Autodesk Inventor part; units mm, degrees
ref_plane "YZ Plane" through (0, 0, 0) normal (1, 0, 0) x (0, 1, 0)
ref_plane "XZ Plane" through (0, 0, 0) normal (0, 1, 0) x (-1, 0, 0)
ref_plane "XY Plane" through (0, 0, 0) normal (0, 0, 1) x (1, 0, 0)
sketch "Sketch1" plane through (0, 0, 0) normal (0, 1, 0) x (-1, 0, 0)
  line L0 (0, 0) -> (50.8, 0)
  line L1 (50.8, 0) -> (50.8, -101.6)
  line L2 (50.8, -101.6) -> (0, -101.6)
  line L3 (0, -101.6) -> (0, 0)
  dimension "d0" = 50.8
  dimension "d1" = 101.6
extrude "Extrusion1" add sketch "Sketch1" along normal blind 3.175
sketch "Sketch2" plane through (0, 0, 0) normal (0, -1, 0) x (1, 0, 0)
  line L0 (-50.8, 0) -> (0, 0)
  line L1 (0, 0) -> (3.175, 0)
  line L2 (3.175, 0) -> (3.175, 3.175)
  line L3 (3.175, 3.175) -> (0, 3.175)
  line L4 (0, 3.175) -> (0, 0)
  line L5 (0, -101.6) -> (-50.8, -101.6)
  line L6 (-50.8, -101.6) -> (-53.975, -101.6)
  line L7 (-53.975, -101.6) -> (-53.975, -104.775)
  line L8 (-53.975, -104.775) -> (-50.8, -104.775)
  line L9 (-50.8, -104.775) -> (-50.8, -101.6)
  line L10 (3.175, 3.175) -> (-53.975, 3.175)
  line L11 (-53.975, 3.175) -> (-53.975, -104.775)
  line L12 (-53.975, -104.775) -> (3.175, -104.775)
  line L13 (3.175, -104.775) -> (3.175, 3.175)
  line L14 (-50.8, -101.6) -> (0, -101.6)
  line L15 (0, -101.6) -> (0, 0)
  line L16 (0, 0) -> (-50.8, 0)
  line L17 (-50.8, 0) -> (-50.8, -101.6)
  dimension "d4" = 3.175
  dimension "d5" = 3.175
  dimension "d6" = 3.175
  dimension "d7" = 3.175
extrude "Extrusion2" add sketch "Sketch2" against normal blind 41.275 contours L17 L6 L11 L10 L4 L0 | L4 L3 L2 L1 | L1 L13 L12 L9 L5 L15 | L9 L8 L7 L6
sketch "Sketch3" plane through (0, 0, 0) normal (0, -1, 0) x (1, 0, 0)
  line L0 (0, -101.6) -> (0, 0)
  line L1 (3.175, 3.175) -> (3.175, -104.775)
  line L2 (0, 0) -> (3.175, 0)
  line L3 (3.175, 0) -> (12.065, 0)
  line L4 (12.065, 0) -> (12.065, -8.89)
  line L5 (12.065, -8.89) -> (3.175, -8.89)
  line L6 (3.175, -8.89) -> (3.175, 0)
  line L7 (-53.975, -104.775) -> (-53.975, 3.175)
  line L8 (-53.975, 0) -> (-62.865, 0)
  line L9 (-62.865, 0) -> (-62.865, -8.89)
  line L10 (-62.865, -8.89) -> (-53.975, -8.89)
  line L11 (-53.975, -8.89) -> (-53.975, 0)
  line L12 (-53.975, -101.6) -> (-62.865, -101.6)
  line L13 (-62.865, -101.6) -> (-62.865, -92.71)
  line L14 (-62.865, -92.71) -> (-53.975, -92.71)
  line L15 (-53.975, -92.71) -> (-53.975, -101.6)
  line L16 (3.175, -101.6) -> (12.065, -101.6)
  line L17 (12.065, -101.6) -> (12.065, -92.71)
  line L18 (12.065, -92.71) -> (3.175, -92.71)
  line L19 (3.175, -92.71) -> (3.175, -101.6)
  dimension "d11" = 8.89
  dimension "d12" = 8.89
  dimension "d13" = 8.89
  dimension "d14" = 8.89
  dimension "d15" = 8.89
  dimension "d16" = 8.89
  dimension "d17" = 8.89
  dimension "d18" = 8.89
extrude "Extrusion3" add sketch "Sketch3" against normal blind 3.175
fillet "Fillet1" radius 3.175 16 edges at (3.175, 1.5875, 0) (12.065, 1.5875, 0) (12.065, 1.5875, -8.89) (3.175, 1.5875, -8.89) (12.065, 1.5875, -92.71) (3.175, 1.5875, -92.71) (12.065, 1.5875, -101.6) (3.175, 1.5875, -101.6) (-53.975, 1.5875, -101.6) (-62.865, 1.5875, -101.6) (-62.865, 1.5875, -92.71) (-53.975, 1.5875, -92.71) (-53.975, 1.5875, 0) (-62.865, 1.5875, 0) (-62.865, 1.5875, -8.89) (-53.975, 1.5875, -8.89)
sketch "Sketch4" plane through (0, 3.175, 0) normal (0, 1, 0) x (1, 0, 0)
  line L0 (-59.69, 8.89) -> (-57.15, 8.89) construction
  line L1 (-58.42, 8.89) -> (-58.42, 0) construction
  line L2 (-59.69, 0) -> (-57.15, 0) construction
  line L3 (6.35, 8.89) -> (8.89, 8.89) construction
  line L4 (7.62, 8.89) -> (7.62, 0) construction
  line L5 (8.89, 0) -> (6.35, 0) construction
  line L6 (8.89, 101.6) -> (6.35, 101.6) construction
  line L7 (7.62, 101.6) -> (7.62, 92.71) construction
  line L8 (6.35, 92.71) -> (8.89, 92.71) construction
  line L9 (-57.15, 101.6) -> (-59.69, 101.6) construction
  line L10 (-58.42, 101.6) -> (-58.42, 92.71) construction
  line L11 (-59.69, 92.71) -> (-57.15, 92.71) construction
  point P0 (0, 0)
  point P1 (-58.42, 97.155)
  point P2 (7.62, 97.155)
  point P3 (7.62, 4.445)
  point P4 (-58.42, 4.445)
hole "Hole1" at (-58.42, 3.175, -97.155) at (7.62, 3.175, -97.155) at (7.62, 3.175, -4.445) at (-58.42, 3.175, -4.445) direction (0, -1, 0) diameter 3.175 depth 25.4 tip angle 118
sketch "Sketch5" plane through (0, 41.275, 0) normal (0, 1, 0) x (1, 0, 0)
  line L0 (-53.975, 104.775) -> (3.175, 104.775)
  line L1 (3.175, 104.775) -> (-9.525, 104.775)
  arc A0 (3.175, 104.775) -> (6.35, 101.6) centre (6.35, 104.775) ccw
  line L2 (3.175, 104.775) -> (3.175, 92.075)
  line L3 (3.175, 92.075) -> (-9.525, 104.775)
  line L4 (3.175, -3.175) -> (-53.975, -3.175)
  line L5 (3.175, -3.175) -> (3.175, 9.525)
  line L6 (3.175, -3.175) -> (3.175, 12.065)
  line L7 (3.175, -3.175) -> (-9.525, -3.175)
  line L8 (-9.525, -3.175) -> (3.175, 9.525)
  line L9 (-25.4, 104.775) -> (-25.4, -3.175) construction
  line L10 (3.175, 104.775) -> (-53.975, 104.775)
  line L11 (-53.975, 104.775) -> (-41.275, 104.775)
  line L12 (-53.975, 104.775) -> (-53.975, 92.075)
  line L13 (-53.975, 92.075) -> (-41.275, 104.775)
  line L14 (-53.975, -3.175) -> (3.175, -3.175)
  line L15 (-53.975, -3.175) -> (-53.975, 9.525)
  line L16 (-53.975, -3.175) -> (-41.275, -3.175)
  line L17 (-41.275, -3.175) -> (-53.975, 9.525)
  point P0 (0, 0)
  dimension "d29" = 12.7
  dimension "d30" = 12.7
  dimension "d31" = 12.7
  dimension "d32" = 12.7
extrude "Extrusion4" add sketch "Sketch5" against normal blind 39.37
fillet "Fillet2" radius 3.175 8 edges at (-6.35, 22.225, -101.6) (0, 22.225, -95.25) (-44.45, 22.225, -101.6) (-50.8, 22.225, -95.25) (-50.8, 22.225, -6.35) (-44.45, 22.225, 0) (-6.35, 22.225, 0) (0, 22.225, -6.35)
sketch "Sketch6" plane through (0, 41.275, 0) normal (0, 1, 0) x (1, 0, 0)
  line L0 (-50.8, 93.9349) -> (-50.8, 7.6651)
  line L1 (0, 0) -> (0, 93.9349)
  point P0 (-50.8, 0)
  point P1 (-50.8, 101.6)
  point P2 (-50.8, 101.6)
  point P3 (0, 101.6)
hole "Hole2" at (0, 41.275, 0) at (-50.8, 41.275, 0) at (-50.8, 41.275, -101.6) at (0, 41.275, -101.6) direction (0, -1, 0) diameter 3.175 depth 9.525 tip angle 118
sketch "Sketch7" plane through (-53.975, 41.275, 3.175) normal (0, 0, 1) x (1, 0, 0)
  line L0 (46.3099, -38.1) -> (10.8401, -38.1) construction
  line L1 (28.575, -38.1) -> (28.575, -31.75) construction
  line L2 (28.575, -31.75) -> (25.4, -31.75) construction
  line L3 (28.575, -31.75) -> (31.75, -31.75) construction
  circle A0 centre (25.4, -31.75) radius 3.175
  circle A1 centre (31.75, -31.75) radius 3.175
  line L4 (25.4, -28.575) -> (31.75, -28.575)
  line L5 (25.4, -34.925) -> (31.75, -34.925)
  point P0 (53.975, -41.275)
  dimension "d49" = 6.35
  dimension "d50" = 3.175
  dimension "d51" = 3.175
  dimension "d52" = 6.35
  dimension "d53" = 6.35
extrude "Extrusion5" cut sketch "Sketch7" against normal blind 25.4
properties part number "box"
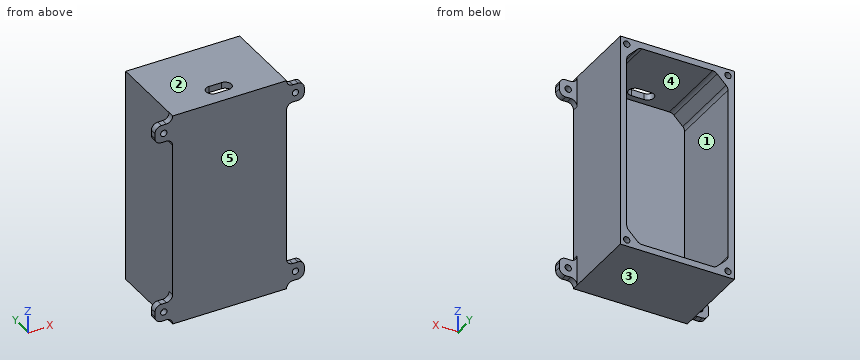
Geometry: final body of the model. Coordinates: model frame, mm. Face numbers are marked on the shaded views. A direction names the side the tool comes from. Round coordinates to 2 decimals unless told otherwise and drop trailing zeros. Write each loop counter-clockwise with the first axis right and the second up, starting at its lowest first coordinate (ties: lowest second). Pieces come first, ordered by that corner, then holes. Notation, with made-up numbers: (-8, 12.5) -> (47, 12.5) arc R15 ccw to (47, 31.5) -> close; hole circle Ø10 at (12, 24.25). An arc over 180 degrees is marked (long way). Use CSV: the item, a comma, the result in double quotes. Start each with the question number.
Q1. Pull-direction query (Z, two-part tool) for the marked faces 1, 2 and 3; classes: pulls with the +Z half, pulls with the -Z half, needs draft (parallel to the pull), parting line crosses it, or undercut.
Q2. Reachability of the marked faces 4 and 5 from +Z, -Z, +X, -X, +Y, -Y: full face, straight path, thin tool, end or side. Return the list, or none.
Q3. Section C-C (z = -20.5). Return loops of the section in (x, y) (3 decimals).
Q4. Section D-D (x = -38.5). Return loops of the section in (y, z) (3 decimals).
Q5. Section A-A (x = -58.42). Return loops of the section in (y, z) (1 decimal), plus the area to 3 significant figures.
Q6. Section B-B (y = 28). Return loops of the section in (x, z) (3 decimals).
Q7. Line query: L1, parallel to Z at x = 7.62, y = 0.7; L2, parallel to Z at x = -15, y = 8.5 (3 decimals); L3, parallel to X at y = 10.5, z = -72.5 (3 decimals). Output: solid intervals per line, ascending.
Q8. First-contact query: pin 1 Ø3 at (y, z) = (13, -65) entering from +X (3 decimals); pin 2 Ø2 at (x, y) = (7, 2) entering from -Z; pin 3 Ø5 at (x, z) = (7.62, -97.155) entering from +Y (3 decimals). Flat tips, straight axial feed; report the tip coordinate or a pass-through.
Result sheet:
1,face 1,"undercut"
1,face 2,"pulls with the +Z half"
1,face 3,"pulls with the -Z half"
2,face 4,"+Y"
2,face 5,"+Z, -Z, +X, -X, -Y"
3,outline,"(-53.975, 0) -> (3.175, 0) -> (3.175, 41.275) -> (0, 41.275) -> (0, 3.175) -> (-50.8, 3.175) -> (-50.8, 41.275) -> (-53.975, 41.275) -> close"
4,outline,"(0, -104.775) -> (41.275, -104.775) -> (41.275, -101.6) -> (3.175, -101.6) -> (3.175, 0) -> (41.275, 0) -> (41.275, 3.175) -> (0, 3.175) -> close"
5,outline,"(0, -101.6) -> (3.2, -101.6) -> (3.2, -98.7) -> (0, -98.7) -> close; (0, -95.6) -> (3.2, -95.6) -> (3.2, -92.7) -> (0, -92.7) -> close; (0, -8.9) -> (3.2, -8.9) -> (3.2, -6) -> (0, -6) -> close; (0, -2.9) -> (3.2, -2.9) -> (3.2, 0) -> (0, 0) -> close"
5,area,"36.3 mm²"
6,outline,"(-53.975, -104.775) -> (3.175, -104.775) -> (3.175, 3.175) -> (-53.975, 3.175) -> close; hole (-50.8, -93.935) arc R3.175 ccw to (-49.87, -96.18) -> (-45.38, -100.67) arc R3.175 ccw to (-43.135, -101.6) -> (-7.665, -101.6) arc R3.175 ccw to (-5.42, -100.67) -> (-0.93, -96.18) arc R3.175 ccw to (0, -93.935) -> (0, -7.665) arc R3.175 ccw to (-0.93, -5.42) -> (-5.42, -0.93) arc R3.175 ccw to (-7.665, 0) -> (-43.135, 0) arc R3.175 ccw to (-45.38, -0.93) -> (-49.87, -5.42) arc R3.175 ccw to (-50.8, -7.665) -> close"
7,L1,"-101.6 to -98.74, -95.57 to -92.71, -8.89 to -6.03, -2.86 to 0"
7,L2,"-104.775 to -101.6, 0 to 3.175"
7,L3,"-53.975 to -50.8, 0 to 3.175"
8,pin 1,"x = 3.175"
8,pin 2,"z = -101.62"
8,pin 3,"y = 3.175"
